CAD build for the part. Positions are in the model's coordinates, mm. Face numbers are marked on the shaded views. A direction names the side the tool comes from. Give positions to 0.01 mm unless a question says otherwise; leave off trailing zeros. Loops run counter-clockwise (first coordinate to the right, second up) from the corner with the lowest first, then second, coordinate; pieces in that order, holes last. Notation, with made-up numbers: M -13.75,33 L 2.25,33 A13 ccw 2.25,54 Z; hole C 58.5,46 d11. An arc over 180 degrees is marked long. One line per question, with ' | ' between items.
```python
from build123d import *

# Parameters (mm, degrees)
SKETCH1_W                       = 65
SKETCH1_H                       = 70
BOSS_EXTRUDE1_DEPTH             = 3
BOSS_EXTRUDE2_DEPTH             = 3
LPATTERN1_COUNT                 = 2
LPATTERN1_PITCH                 = 67
BOSS_EXTRUDE3_REACH             = 77.771
SKETCH4_W                       = 19
SKETCH4_H                       = 11
FILLET4_R                       = 2
FILLET3_R                       = 1.5
F_8_0MM_DOWEL_HOLE1_D           = 8
F_8_0MM_DOWEL_HOLE1_CSINK_D     = 8.05
F_8_0MM_DOWEL_HOLE1_CSINK_ANGLE = 90
F_1_0_26_DIAMETER_HOLE1_D       = 26
LPATTERN2_COUNT                 = 2
LPATTERN2_PITCH                 = 27


with BuildPart() as part:
    # Sketch1 → Boss-Extrude1 (new body)
    with BuildSketch(Plane.XY):
        Rectangle(SKETCH1_W, SKETCH1_H)
    extrude(amount=BOSS_EXTRUDE1_DEPTH)

    # Sketch2 → Boss-Extrude2 (add)
    with BuildSketch(Plane(origin=(-2.5, 35, 0), x_dir=(0, 0, -1), z_dir=(0, 1, 0))):
        Polygon((-14, -0.5), (-14, 30), (-3, 30), (-3, -35), (-8, -35), align=None)
    boss_extrude2 = extrude(amount=-BOSS_EXTRUDE2_DEPTH)

    # LPattern1: Boss-Extrude2 ×2
    with Locations(*[(0, -i * LPATTERN1_PITCH, 0) for i in range(1, LPATTERN1_COUNT)]):
        add(boss_extrude2)

    # Sketch4 → Boss-Extrude3 (add, up to next)
    with BuildSketch(Plane.XZ.offset(-32), mode=Mode.PRIVATE) as boss_extrude3_sk1:
        with Locations((-23, 8.5)):
            Rectangle(SKETCH4_W, SKETCH4_H)
    boss_extrude3_tool1 = extrude(boss_extrude3_sk1.sketch, amount=BOSS_EXTRUDE3_REACH, mode=Mode.PRIVATE) - part.part
    add(boss_extrude3_tool1.solids().sort_by_distance((-23, 32, 8.5))[0])

    # Fillet4
    fillet4_edges = [part.edges().sort_by_distance(p)[0] for p in [
        (32.5, 33.5, 8),
        (32.5, -33.5, 8),
    ]]
    fillet(fillet4_edges, radius=FILLET4_R)

    # Fillet3
    fillet3_edges = [part.edges().sort_by_distance(p)[0] for p in [
        (14.421341175, 32, 11.144114578),
        (14.421341175, 35, 11.144114578),
        (-17.25, 35, 14),
        (-7.75, 32, 14),
        (14.421341175, -32, 11.144114578),
        (-7.75, -32, 14),
        (-17.25, -35, 14),
        (14.421341175, -35, 11.144114578),
        (32.5, 32, 4.658902823),
        (32.030582356, 32, 7.605174145),
        (32.5, 35, 3.158902823),
        (32.030582356, 35, 7.605174145),
        (32.5, -32, 4.658902823),
        (32.030582356, -32, 7.605174145),
        (32.5, -35, 3.158902823),
        (32.030582356, -35, 7.605174145),
    ]]
    fillet(fillet3_edges, radius=FILLET3_R - 0.0001)  # a hair under: the kernel refuses the full size

    # Ø8.0mm Dowel Hole1 (through all)
    with Locations(Plane.ZY.offset(32.5)):
        with Locations((7, 0)):
            CounterSinkHole(F_8_0MM_DOWEL_HOLE1_D / 2, F_8_0MM_DOWEL_HOLE1_CSINK_D / 2, counter_sink_angle=F_8_0MM_DOWEL_HOLE1_CSINK_ANGLE)

    # Ø1.0 (26) Diameter Hole1 (through all)
    with Locations(Plane.XY.offset(3)):
        with Locations((5.5, -14.5)):
            f_1_0_26_diameter_hole1 = Hole(F_1_0_26_DIAMETER_HOLE1_D / 2)

    # LPattern2: Ø1.0 (26) Diameter Hole1 ×2
    with Locations(*[(0, i * LPATTERN2_PITCH, 0) for i in range(1, LPATTERN2_COUNT)]):
        add(f_1_0_26_diameter_hole1, mode=Mode.SUBTRACT)


solid = part.part
```
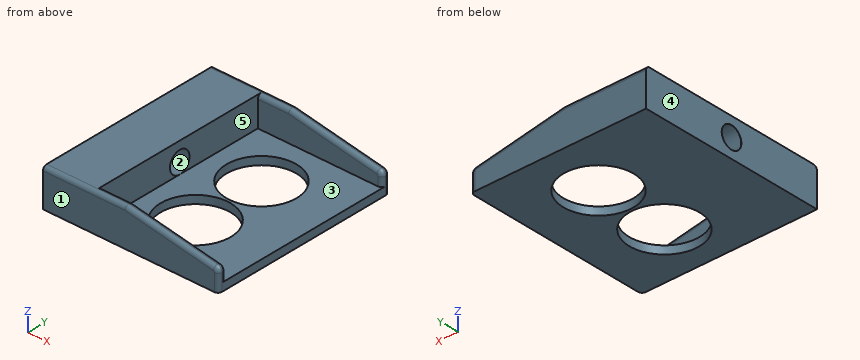
Item 1: Saw through at A-A on y = -14.5. Give the cut face in (x, z), and give its area (3 significant figures).
Conclusion:
outline: M -32.5,0 L -7.5,0 L -7.5,3 L -13.5,3 L -13.5,14 L -32.5,14 Z; M 18.5,0 L 32.5,0 L 32.5,3 L 18.5,3 Z | area: 326 mm²
Item 2: Drill centre lines: line 1 along Y through (x, z) = (5.5, 1.2); line 2 along Z through (x, y) = (-21, 0); line 3 along Y through (x, z) = (-22, 6.75). Where is each one in solid material? Low to high. Write a range as [from, to].
Conclusion:
line 1: [-35, -27.5], [-1.5, -0.5], [25.5, 35] | line 2: [0, 3], [11, 14] | line 3: [-35, -3.99], [3.99, 35]
Item 3: Saw through at B-B on x = -20. Give the cut face in (y, z).
Conclusion:
outline: M -35,0 L 35,0 L 35,12.5 A1.5 ccw 33.5,14 L -33.5,14 A1.5 ccw -35,12.5 Z; hole C 0,7 d8
Item 4: Mould opens along Z. For the marked faces 1, 2 and 3 say: pulls with the +Z half, pulls with the -Z half, needs draft (parallel to the pull), parting line crosses it, or undercut.
Conclusion:
face 1: needs draft | face 2: undercut | face 3: pulls with the +Z half
Item 5: Saw through at D-D on y = 17. Give the cut face in (x, z).
Conclusion:
outline: M -32.5,0 L -6.7,0 L -6.7,3 L -13.5,3 L -13.5,14 L -32.5,14 Z; M 17.7,0 L 32.5,0 L 32.5,3 L 17.7,3 Z
Item 6: Drop flat-ended pins along their axis: P1, Ø5, axis at x = 13.5, z = 10, coming from the -Y side; P2, Ø3.5, axis at y = 9.5, z = 8.5, coming from the +X side; P3, Ø1, axis at x = 9.5, y = -26.5, coming from the +Z side. Give the stop position or say it passes through.
Conclusion:
P1: y = -35 | P2: x = -13.5 | P3: z = 3
Item 7: Saw through at C-C on x = 6.5. State how many separate pieces and enclosed holes the cut face has, and give its area (3 significant figures).
Conclusion:
separate pieces: 3 | enclosed holes: 0 | area: 110 mm²
Item 8: 3-axis set-ups, long thin cutter, end or side, ignore diameter. For the marked faces 4 and 5: which of +Z, -Z, +X, -X, +Y, -Y reach the whole face in a straight line?
Conclusion:
face 4: +Z, -Z, -X, +Y, -Y | face 5: +Z, +X
